Design review of the part built by this model. Coordinates are the model's own, in mm. Face numbers are marked on the shaded views. A direction names the side the tool comes from. Round coordinates to 2 decimals unless told otherwise and drop trailing zeros. Loops run counter-clockwise (first coordinate to the right, second up) from the corner with the lowest first, then second, coordinate; pieces in that order, holes last. Notation, with made-up numbers: (10, 87.25) - (26, 87.25) arc R24 ccw to (26, 99.25) - close; hole circle Ø2 at (27.25, 54). An arc over 180 degrees is marked (long way). Return JSON: item names as keys, results as strings. Group by question number.
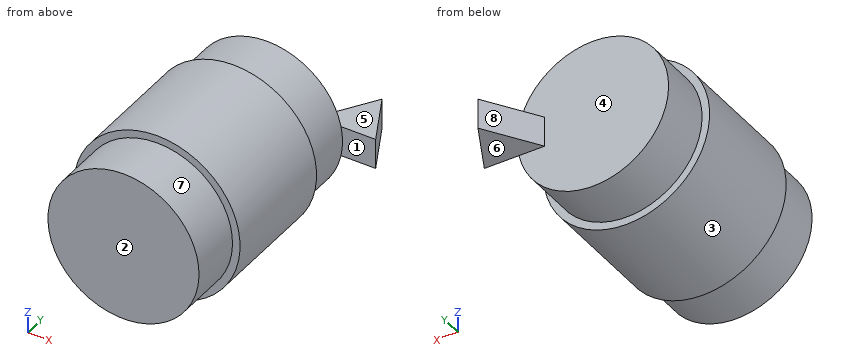
from build123d import *

# Parameters (mm, degrees)
SKETCH_1_R      = 5
EXTRUDE_1_DEPTH = 7.5
SKETCH_2_R      = 5.5
EXTRUDE_2_DEPTH = 4
EXTRUDE_3_DEPTH = 1
SCALE_1_SCALE   = 3
SCALE_2_SCALE   = 0.7


with BuildPart() as part:
    # 草图1 → 凸台-拉伸1 (new, symmetric)
    with BuildSketch(Plane(origin=(0, 0, 0), x_dir=(1, 0, 0), z_dir=(0, 1, 0))):
        with Locations(Location((0, 0, 0), (0, 0, 270))):
            Circle(SKETCH_1_R)
    extrude(amount=EXTRUDE_1_DEPTH, both=True)

    # 草图2 → 凸台-拉伸2 (add, symmetric)
    with BuildSketch(Plane(origin=(0, 0, 0), x_dir=(1, 0, 0), z_dir=(0, 1, 0))):
        with Locations(Location((0, 0, 0), (0, 0, 270))):
            Circle(SKETCH_2_R)
    extrude(amount=EXTRUDE_2_DEPTH, both=True)

    # 草图3 → 凸台-拉伸3 (add, symmetric)
    with BuildSketch(Plane.XY):
        Polygon((3.208751117, 7.5), (7.19369463, 7.5), (5.433428229, 10.94766776), align=None)
    extrude(amount=EXTRUDE_3_DEPTH, both=True)


with BuildPart() as part_1:
    # 缩放比例1: scaled about (0.054783729, 0.089765176, 0)
    add(part.part.scale(SCALE_1_SCALE).moved(Location((-0.109567458, -0.179530352, 0))))


with BuildPart() as part_2:
    # 缩放比例2: scaled about (0.05478373, 0.089765175, 0)
    add(part_1.part.scale(SCALE_2_SCALE).moved(Location((0.016435119, 0.026929553, 0))))


solid = part_2.part
Q1. Insertion check: pin 1 Ø12 at (y, z) = (9.5, -7.5) entering from +X; pin 2 Ø7 at (x, z) = (-2, 3) entering from +Y; pin 3 Ø6 at (x, y) = (10.5, 19.5) entering from +Z. Each pin has a flat end and moves straight along its axis. Give the tip position at first contact, or say it passes through.
Q2. Add section B-B, the plane x = -7.5. State the section outline as (y, z) points.
Q3. Tool access review of the marked faces 5, 6, 7 and 8: name each direction out of +Z, -Z, +X, -X, +Y, -Y from which nothing blocks a thin tool from reaching the whole face with its end or side.
Q4. Add section C-C, the plane y = 13.5. State the section outline as (x, z) points.
Q5. For line 1 (Y direction, x = 7.25, z = 8); line 2 (Y direction, x = 0.75, z = 0); line 3 (X direction, y = 10, z = -0.25), list the stretches that pass through material, from the lowest coordinate up.
Q6. Draft analysis for pull direction Y (two halves, no side actions). For the marked faces 1, 2, 3 and 4, state which applies: pulls with the +Y half, pulls with the -Y half, needs draft (parallel to the pull), parting line crosses it, or undercut.
Q7. Add section A-A, the plane z = 0. State the section outline as (x, y) points, plus the area to 3 significant figures.
Q8. Add section D-D, the plane z = 6. State the section outline as (x, y) points.
Evaluation:
{
 "1": {"pin 1": "x = 11.38", "pin 2": "y = 15.65", "pin 3": "z = 2.1"},
 "2": {"outline": "(-15.85, -7.41) - (-8.5, -7.41) - (-8.5, -8.83) - (8.3, -8.83) - (8.3, -7.41) - (15.65, -7.41) - (15.65, 7.41) - (8.3, 7.41) - (8.3, 8.83) - (-8.5, 8.83) - (-8.5, 7.41) - (-15.85, 7.41) - close"},
 "3": {"face 5": "+Z, +X, -X, +Y", "face 6": "-Z, +X, -X, +Y", "face 7": "-Y", "face 8": "+Z, -Z, -X, +Y"},
 "4": {"outline": "circle Ø21 at (-0.06, 0)"},
 "5": {"line 1": "-8.5 to 8.3", "line 2": "-15.85 to 15.65", "line 3": "-10.56 to 10.44"},
 "6": {"face 1": "undercut", "face 2": "pulls with the -Y half", "face 3": "needs draft", "face 4": "pulls with the +Y half"},
 "7": {"outline": "(-11.61, -8.5) - (-10.56, -8.5) - (-10.56, -15.85) - (10.44, -15.85) - (10.44, -8.5) - (11.49, -8.5) - (11.49, 8.3) - (10.44, 8.3) - (10.44, 15.65) - (15.05, 15.65) - (11.35, 22.89) - (6.68, 15.65) - (-10.56, 15.65) - (-10.56, 8.3) - (-11.61, 8.3) - close", "area": "727 mm²"},
 "8": {"outline": "(-9.93, -8.5) - (-8.68, -8.5) - (-8.68, -15.85) - (8.56, -15.85) - (8.56, -8.5) - (9.81, -8.5) - (9.81, 8.3) - (8.56, 8.3) - (8.56, 15.65) - (-8.68, 15.65) - (-8.68, 8.3) - (-9.93, 8.3) - close"}
}
